Autodesk Inventor part; units mm, degrees
ref_plane "YZ Plane" through (0, 0, 0) normal (1, 0, 0) x (0, 1, 0)
ref_plane "XZ Plane" through (0, 0, 0) normal (0, 1, 0) x (-1, 0, 0)
ref_plane "XY Plane" through (0, 0, 0) normal (0, 0, 1) x (1, 0, 0)
sketch "Sketch1" plane through (0, 0, 0) normal (0, 0, 1) x (1, 0, 0)
  line L0 (-28.2731, 30.1639) -> (-44.2731, 30.1639)
  arc A0 (11.7269, 37.1639) -> (6.7269, 42.1639) centre (6.7269, 37.1639) ccw
  line L1 (-23.2731, 42.1639) -> (6.7269, 42.1639)
  arc A1 (-23.2731, 42.1639) -> (-28.2731, 37.1639) centre (-23.2731, 37.1639) ccw
  line L2 (-28.2731, 30.1639) -> (-28.2731, 37.1639)
  line L3 (-28.2731, 30.1639) -> (-44.2731, 30.1639)
  arc A2 (-44.2731, 30.1639) -> (-49.2731, 25.1639) centre (-44.2731, 25.1639) ccw
  line L4 (-49.2731, 25.1639) -> (-49.2731, -25.1361)
  arc A3 (-49.2731, -25.1361) -> (-44.2731, -30.1361) centre (-44.2731, -25.1361) ccw
  line L5 (-44.2731, -30.1361) -> (-28.2731, -30.1361)
  line L6 (-28.2731, -30.1361) -> (-28.2731, -37.1361)
  arc A4 (-28.2731, -37.1361) -> (-23.2731, -42.1361) centre (-23.2731, -37.1361) ccw
  line L7 (-23.2731, -42.1361) -> (6.7269, -42.1361)
  arc A5 (6.7269, -42.1361) -> (11.7269, -37.1361) centre (6.7269, -37.1361) ccw
  line L8 (11.7269, -37.1361) -> (11.7269, -30.1361)
  line L9 (11.7269, -30.1361) -> (27.7269, -30.1361)
  arc A6 (27.7269, -30.1361) -> (32.7269, -25.1361) centre (27.7269, -25.1361) ccw
  line L10 (32.7269, -25.1361) -> (32.7269, 25.1639)
  arc A7 (32.7269, 25.1639) -> (27.7269, 30.1639) centre (27.7269, 25.1639) ccw
  line L11 (27.7269, 30.1639) -> (11.7269, 30.1639)
  line L12 (11.7269, 37.1639) -> (11.7269, 30.1639)
  line L13 (1.7269, 36.9139) -> (1.7269, 33.9139)
  line L14 (1.7269, 33.9139) -> (-0.2731, 33.9139)
  line L15 (-0.2731, 33.9139) -> (-0.2731, 36.9139)
  line L16 (-0.2731, 36.9139) -> (1.7269, 36.9139)
  line L17 (-16.2731, 36.9139) -> (-16.2731, 33.9139)
  line L18 (-16.2731, 33.9139) -> (-18.2731, 33.9139)
  line L19 (-18.2731, 33.9139) -> (-18.2731, 36.9139)
  line L20 (-18.2731, 36.9139) -> (-16.2731, 36.9139)
  line L21 (-3.7731, 36.9139) -> (-3.7731, 33.9139)
  line L22 (-3.7731, 33.9139) -> (-12.7731, 33.9139)
  line L23 (-12.7731, 33.9139) -> (-12.7731, 36.9139)
  line L24 (-12.7731, 36.9139) -> (-3.7731, 36.9139)
  line L25 (1.7269, -33.8861) -> (1.7269, -36.8861)
  line L26 (1.7269, -36.8861) -> (-0.2731, -36.8861)
  line L27 (-0.2731, -36.8861) -> (-0.2731, -33.8861)
  line L28 (-0.2731, -33.8861) -> (1.7269, -33.8861)
  line L29 (-16.2731, -33.8861) -> (-16.2731, -36.8861)
  line L30 (-16.2731, -36.8861) -> (-18.2731, -36.8861)
  line L31 (-18.2731, -36.8861) -> (-18.2731, -33.8861)
  line L32 (-18.2731, -33.8861) -> (-16.2731, -33.8861)
  line L33 (-3.7731, -33.8861) -> (-3.7731, -36.8861)
  line L34 (-3.7731, -36.8861) -> (-12.7731, -36.8861)
  line L35 (-12.7731, -36.8861) -> (-12.7731, -33.8861)
  line L36 (-12.7731, -33.8861) -> (-3.7731, -33.8861)
  circle A8 centre (10.1389, 23.4843) radius 1.6
  circle A9 centre (-40.6611, 8.2443) radius 1.6
  circle A10 centre (-40.6611, -19.6957) radius 1.6
  circle A11 centre (11.4089, -24.7757) radius 1.6
  point P0 (0, 0)
extrude "Extrusion1" add sketch "Sketch1" along normal blind 3
properties part number "base2protopress"
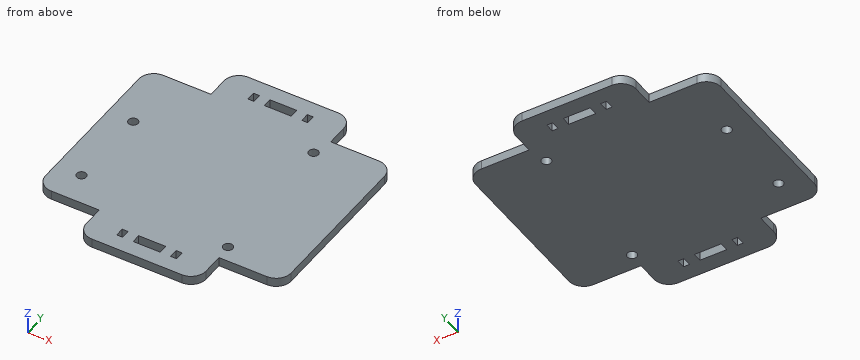
Input: part model. Units: mm. Frame: model coordinates. Coordinates: 2 decimals unless noted, no trailing zeros. Loops run counter-clockwise (first coordinate to the right, second up) from the corner with the lowest first, then second, coordinate; pieces in that order, holes last. Notation, with made-up numbers: M 70,79.5 L 94,79.5 A29 cw 94,109.5 Z; hole C 15,-25.5 d1. An arc over 180 degrees is marked long. Use a Markdown table: item, result. Add a question column.
1) Pin query (flat end, axial travel): P1, Ø2.5, axis at x = -40.66, y = -19.7, coming from the +Z side; P2, Ø0.9, axis at y = -34, z = 1.5, coming from the +X side; P3, Ø1.5, axis at y = 35.5, z = 1, coming from the -X side. Return the tip coordinate at first contact, or that it passes through.
2) Section C-C, the plane z = 2.35. Give the number of separate pieces and of enclosed holes in the cut face, plus the area to 3 significant figures.
3) Section B-B, the plane x = 21. Return the cut outline in (y, z).
4) Section A-A, the plane x = -7. Return the cut outline in (y, z).
5) Line query: L1, parallel to Y at x = -18, z = 1.9; L2, parallel to Y at x = 10.5, z = 1.8; L3, parallel to X at y = -20, z = 1.95. Output: solid intervals per line, ascending. Write a range as from..to.
Answer below:
| question | item | result |
|---|---|---|
| 1 | P1 | through |
| 1 | P2 | x = 11.73 |
| 1 | P3 | x = -28.27 |
| 2 | separate pieces | 1 |
| 2 | enclosed holes | 10 |
| 2 | area | 5,750 mm2 |
| 3 | outline | M -30.14,0 L 30.16,0 L 30.16,3 L -30.14,3 Z |
| 4 | outline | M -42.14,0 L -36.89,0 L -36.89,3 L -42.14,3 Z; M -33.89,0 L 33.91,0 L 33.91,3 L -33.89,3 Z; M 36.91,0 L 42.16,0 L 42.16,3 L 36.91,3 Z |
| 5 | L1 | -42.14..-36.89, -33.89..33.91, 36.91..42.16 |
| 5 | L2 | -40.42..-26.09, -23.46..21.93, 25.04..40.44 |
| 5 | L3 | -49.27..-42.23, -39.09..32.73 |
